```python
from build123d import *

# Parameters (mm, degrees)
MODEL_R                 = 8
SALIENTE_EXTRUIR1_DEPTH = 0.1


with BuildPart() as part:
    # Model → Saliente-Extruir1 (new body)
    with BuildSketch(Plane.XY):
        with BuildLine():
            ThreePointArc((27.14548024, 7.194414678), (25.273911912, 20.263089859), (14.523964876, 27.926749411))
            ThreePointArc((14.523964876, 27.926749411), (10.054231622, 29.274256382), (5.841127337, 31.28523691))
            ThreePointArc((5.841127337, 31.28523691), (6.23485784, 18.070799585), (15.423765374, 8.566045203))
            ThreePointArc((15.423765374, 8.566045203), (21.202282113, 7.176560753), (27.14548024, 7.194414678))
        make_face()
        with Locations((16.501428973, 17.994891823)):
            Circle(MODEL_R, mode=Mode.SUBTRACT)
    extrude(amount=SALIENTE_EXTRUIR1_DEPTH)


solid = part.part
```
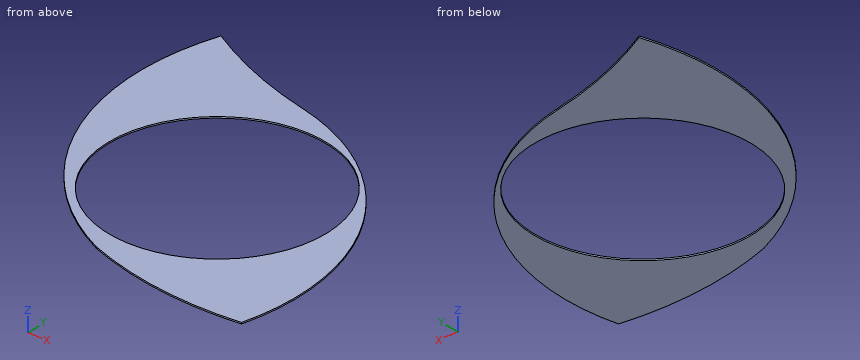
The listing builds one solid part. Answer for the finished solid, in the listing's coordinates (mm). Coordinates: 2 decimals unless noted, no trailing zeros. Order: outer loops, then holes, each group sorted by start corner. A loop starts at its lowest first (then second) coordinate and runs counter-clockwise, first axis right, second up. Notation, with made-up numbers: M 45.25,80 L 84.25,80 A18 cw 84.25,90 Z; hole C 81.25,-31 d10. An arc over 180 degrees is marked long. Answer as a JSON object with one key per item and string values. Group by question number.
1. Straight lines are drawn through the part: line 1 (Y direction, x = 20.5, z = 0.05); line 2 (Y direction, x = 15.75, z = 0.05); line 3 (X direction, y = 17.5, z = 0.05). For each, find the intervals that lie inside material, in ascending order.
2. Section B-B on x = 11.75 is taken. Write down the section's boundary in (y, z).
3. Section D-D on y = 29.5 is taken. Write down the section's boundary in (x, z).
4. Section C-C on z = 0.05 is taken. Write down the section's boundary in (x, y), then the cut area to 3 significant figures.
5. Section A-A on y = 13.5 is taken. Write down the section's boundary in (x, z), then the cut area to 3 significant figures.
Values follow:
{
 "1": {"line 1": "7.27 to 11.07, 24.92 to 25.33", "line 2": "8.45 to 10.03, 25.96 to 27.61", "line 3": "6.49 to 8.52, 24.49 to 26.63"},
 "2": {"outline": "M 10.82,0 L 11.56,0 L 11.56,0.1 L 10.82,0.1 Z; M 24.43,0 L 28.67,0 L 28.67,0.1 L 24.43,0.1 Z"},
 "3": {"outline": "M 5.31,0 L 9.49,0 L 9.49,0.1 L 5.31,0.1 Z"},
 "4": {"outline": "M 5.84,31.29 A18.31 ccw 15.42,8.57 A24.93 ccw 27.15,7.19 A16.77 ccw 14.52,27.93 A30.64 cw Z; hole C 16.5,17.99 d16", "area": "166 mm2"},
 "5": {"outline": "M 9.01,0 L 9.88,0 L 9.88,0.1 L 9.01,0.1 Z; M 23.12,0 L 27.6,0 L 27.6,0.1 L 23.12,0.1 Z", "area": "0.536 mm2"}
}
